```python
from build123d import *

# Parameters (mm, degrees)
F0_R     = 4
F0_R_2   = 2.375
F1_DEPTH = 6
F3_DEPTH = 7.62


with BuildPart() as f1:
    # F0 (on Top) → F1 (new body, symmetric)
    with BuildSketch(Plane.XY):
        Circle(F0_R)
        Circle(F0_R_2, mode=Mode.SUBTRACT)
    extrude(amount=F1_DEPTH, both=True)

    # F2 (on face) → F3 (join)
    with BuildSketch(Plane.XY.offset(6)):
        with BuildLine():
            ThreePointArc((-1.9231746538, -24.0532388516), (-3.7478638442, -13.1853053628), (1.7141412384, -3.614100139))
            ThreePointArc((1.7141412384, -3.614100139), (-1.026790754, -3.8659669874), (-3.2815280129, -2.2872634087))
            ThreePointArc((-3.2815280129, -2.2872634087), (-8.3896329921, -12.8229645422), (-4.4550945329, -23.8507994143))
            Line((-4.4550945329, -23.8507994143), (-1.9231746538, -24.0532388516))
        make_face()
        with BuildLine():
            ThreePointArc((-3.2815280129, -2.2872634087), (-3.9361819774, 0.7116680692), (-2.2728769699, 3.2915088151))
            ThreePointArc((-2.2728769699, 3.2915088151), (-12.6666400466, 8.2098960617), (-23.5180136949, 4.4061434477))
            Line((-23.5180136949, 4.4061434477), (-24.0532388516, 1.9231746538))
            ThreePointArc((-24.0532388516, 1.9231746538), (-12.8963973291, 3.6215266899), (-3.2815280129, -2.2872634087))
        make_face()
        with BuildLine():
            ThreePointArc((1.9231746538, 24.0532388516), (6.2669055314, 13.6088157667), (2.8225517459, 2.8342903241))
            ThreePointArc((2.8225517459, 2.8342903241), (3.6939279219, 1.5345672055), (4, 0))
            ThreePointArc((4, 0), (3.9962376082, -0.17345022), (3.9849575106, -0.3465741462))
            ThreePointArc((3.9849575106, -0.3465741462), (11.1793944272, 12.4572056596), (4.1165925533, 25.3340658962))
            Line((4.1165925533, 25.3340658962), (1.9231746538, 24.0532388516))
        make_face()
        with BuildLine():
            ThreePointArc((24.0532388516, -1.9231746538), (13.7489229147, -4.5738896933), (3.9849575106, -0.3465741462))
            ThreePointArc((3.9849575106, -0.3465741462), (3.2846785483, -2.2827366984), (1.7141412384, -3.614100139))
            ThreePointArc((1.7141412384, -3.614100139), (13.1058972443, -9.3455478814), (24.8347379439, -4.3399616053))
            Line((24.8347379439, -4.3399616053), (24.0532388516, -1.9231746538))
        make_face()
    extrude(amount=-F3_DEPTH)


solid = f1.part
```
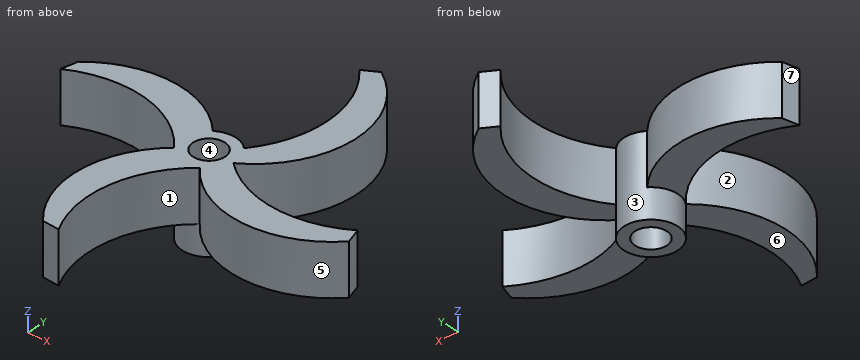
Input: part model. Units: mm. Frame: model coordinates. Face numbers are marked on the shaded views. A direction names the side the tool comes from. Coordinates: 2 decimals unless noted, no trailing zeros. Write each loop counter-clockwise with the first axis right and the second up, starting at its lowest first coordinate (ties: lowest second). Pieces come first, ordered by that corner, then holes. Notation, with made-up numbers: (65, 38.25) -> (100, 38.25) arc R33 cw to (100, 66.25) -> close; hole circle Ø11 at (79.25, 50). An arc over 180 degrees is marked (long way). Answer as a JSON object with one key per item and string values.
1. First-contact query: P1, Ø3, axis at x = -17.5, y = 3.5, coming from the -Z side; P2, Ø5.5, axis at x = 0, y = 0, coming from the +Z side; P3, Ø4, axis at y = 11, z = 3.5, coming from the +X side; P4, Ø3, axis at x = 9, z = 3, coming from the -Y side. Flat tips, straight axial feed; report the tip coordinate or a pass-through.
Result set:
{"P1": "stops at z = -1.62", "P2": "stops at z = 6", "P3": "stops at x = 11.18", "P4": "stops at y = -9.04"}
2. Section C-C on z = -4.75. Return the cut outline in (x, y) (3 decimals).
Result set:
{"outline": "circle Ø8 at (0, 0); hole circle Ø4.75 at (0, 0)"}
3. Section D-D on x = 8. Return the cut outline in (y, z), then the cut area to 3 significant figures.
Result set:
{"outline": "(-8.29, -1.62) -> (-3.04, -1.62) -> (-3.04, 6) -> (-8.29, 6) -> close; (3.26, -1.62) -> (21.81, -1.62) -> (21.81, 6) -> (3.26, 6) -> close", "area": "181 mm2"}
4. Section B-B on y = -5.5. Return the cut outline in (x, z).
Result set:
{"outline": "(-6.03, -1.62) -> (-0.15, -1.62) -> (-0.15, 6) -> (-6.03, 6) -> close; (3.49, -1.62) -> (23.67, -1.62) -> (23.67, 6) -> (3.49, 6) -> close"}
5. Section A-A on x = 0. Return the cut outline in (y, z) (3 decimals).
Result set:
{"outline": "(-5.322, -1.62) -> (-4, -1.62) -> (-4, -6) -> (-2.375, -6) -> (-2.375, 6) -> (-5.322, 6) -> close; (2.375, -6) -> (4, -6) -> (4, 6) -> (2.375, 6) -> close"}
6. Access query for the marked faces 1, 2 and 3. Directions: +Z, -Z, +X, -X, +Y, -Y. A direction counts if a zero-diameter tool reaches every point of the face in a straight line with its end or side. Return the directions, or none.
Result set:
{"face 1": "+Z, -Z", "face 2": "+Z, -Z, -X", "face 3": "-Z"}
7. Material intervals for line 1 (Y direction, x = 0, z = -2.5) (3 decimals); line 2 (Z direction, x = 11.5, y = -5); line 3 (X direction, y = -12, z = 2), sorted ascending. Write a range as from..to.
Result set:
{"line 1": "y = -4..-2.375, 2.375..4", "line 2": "z = -1.62..6", "line 3": "x = -8.32..-3.49"}
8. Mould query, pull axis X, two halves, no side actions, for the marked faces 4, 5, 6 and 7. Classes: released by +X, released by -X, zero draft, split by the parting line, or undercut.
Result set:
{"face 4": "undercut", "face 5": "undercut", "face 6": "zero draft", "face 7": "released by -X"}
